Work out the finished part from the listing and answer in its coordinate system (mm). A direction names the side the tool comes from. Coordinates: 2 decimals unless noted, no trailing zeros. Order: outer loops, then holes, each group sorted by start corner. A loop starts at its lowest first (then second) coordinate and runs counter-clockwise, first axis right, second up.
```python
from build123d import *

# Parameters (mm, degrees)
F0_R     = 37.5
F1_DEPTH = 30
F2_R     = 31.5
F3_DEPTH = 7
F4_R     = 3.1
F5_DEPTH = 23
F6_R     = 18.25
F7_DEPTH = 23
F9_DEPTH = 10


with BuildPart() as f1:
    # F0 (on Top) → F1 (new body)
    with BuildSketch(Plane.XY):
        Circle(F0_R)
    extrude(amount=F1_DEPTH)

    # F2 (on face) → F3 (cut)
    with BuildSketch(Plane(origin=(0, 0, 0), x_dir=(1, 0, 0), z_dir=(0, 0, -1))):
        Circle(F2_R)
    extrude(amount=-F3_DEPTH, mode=Mode.SUBTRACT)

    # F4 (on face) → F5 (cut, through all)
    with BuildSketch(Plane(origin=(0, 0, 7), x_dir=(1, 0, 0), z_dir=(0, 0, -1))):
        with Locations((25, 0)):
            Circle(F4_R)
        with Locations((17.6776695297, 17.6776695297)):
            Circle(F4_R)
        with Locations((0, 25)):
            Circle(F4_R)
        with Locations((-17.6776695297, 17.6776695297)):
            Circle(F4_R)
        with Locations((-25, 0)):
            Circle(F4_R)
        with Locations((-17.6776695297, -17.6776695297)):
            Circle(F4_R)
        with Locations((0, -25)):
            Circle(F4_R)
        with Locations((17.6776695297, -17.6776695297)):
            Circle(F4_R)
    extrude(amount=-F5_DEPTH, mode=Mode.SUBTRACT)

    # F6 (on face) → F7 (cut, through all)
    with BuildSketch(Plane.XY.offset(30)):
        Circle(F6_R)
    extrude(amount=-F7_DEPTH, mode=Mode.SUBTRACT)

    # F8 (on face) → F9 (cut)
    with BuildSketch(Plane.XY.offset(30)):
        with BuildLine():
            Line((-2.9506152383, 18.0098964382), (-10.41284244, 36.0253065541))
            ThreePointArc((-10.41284244, 36.0253065541), (-14.1961717752, 34.7090579954), (-17.8175149302, 32.9967598669))
            Line((-17.8175149302, 32.9967598669), (-10.3702066072, 15.0173671103))
            ThreePointArc((-10.3702066072, 15.0173671103), (-6.8264105945, 16.9252065983), (-2.9506152383, 18.0098964382))
        make_face()
    extrude(amount=-F9_DEPTH, mode=Mode.SUBTRACT)


solid = f1.part
```
1. For faces 4 (the flat face through (-6.63, 26.89, 25.07)), 5 (the flat face through (-8.86, -16.14, 30)), 6 (the flat face through (14, 14, 7)), determine the directions among +Z, -Z, +X, -X, +Y, -Y from which every point of the face is accessible in a straight line to the end or side of a thin tool.
2. The part is cut by section C-C (x = 25). Determine the outline of the cut face in (y, z).
3. The mould has two halves that part along Y. Classify faces 1 (the flat face through (-9, 31, 0)), 2 (the cylindrical face through (-4.88, 37.18, 14.79)), 3 (the cylindrical face through (20.635, -18.609, 18.339)): released by +Y, released by -Y, zero draft, split by the parting line, or undercut.
4. Consider probe 1 along Y at (x, z) = (0, 19.5); probe 2 along Y at (x, z) = (-15.5, 22). Determine where each line is inside the solid, lowest interval first.
5. The part is cut by section A-A (y = 0). Determine the outline of the cut face in (x, z).
6. Flat-ended cylindrical pins translate along their axes: pin 1 (6 mm diameter, centred on x = 24, z = 21.5, fed in from +Y); pin 2 (8 mm diameter, centred on y = -5.5, z = 17, fed in from -X); pin 3 (1.5 mm diameter, centred on x = -21, z = 8.5, fed in from -Y). Find the tip coordinate at first contact, or state that the pin passes through.
7. The part is cut by section D-D (z = 15.25). Count the separate pieces of the cut face and the enclosed holes in it, plus the area to 3 significant figures.
Worked out:
1. face 4: +Z
1. face 5: +Z, +X, -X, +Y, -Y
1. face 6: -Z
2. outline: (-27.95, 0) - (-19.16, 0) - (-19.16, 7) - (-3.1, 7) - (-3.1, 30) - (-27.95, 30) - close; (3.1, 7) - (19.16, 7) - (19.16, 0) - (27.95, 0) - (27.95, 30) - (3.1, 30) - close
3. face 1: zero draft
3. face 2: split by the parting line
3. face 3: undercut
4. probe 1: y = -37.5 to -28.1, -21.9 to -18.25, 18.25 to 21.9, 28.1 to 37.5
4. probe 2: y = -34.15 to -19.88, -15.47 to -9.63, 9.63 to 15.47, 19.88 to 27.4
5. outline: (-37.5, 0) - (-31.5, 0) - (-31.5, 7) - (-28.1, 7) - (-28.1, 30) - (-37.5, 30) - close; (-21.9, 7) - (-18.25, 7) - (-18.25, 30) - (-21.9, 30) - close; (18.25, 7) - (21.9, 7) - (21.9, 30) - (18.25, 30) - close; (28.1, 7) - (31.5, 7) - (31.5, 0) - (37.5, 0) - (37.5, 30) - (28.1, 30) - close
6. pin 1: stops at y = 31.07
6. pin 2: stops at x = -37.47
6. pin 3: stops at y = -31.56
7. separate pieces: 1
7. enclosed holes: 9
7. area: 3,130 mm2
